The listing builds one solid part. Answer for the finished solid, in the listing's coordinates (mm). Face numbers are marked on the shaded views. Round coordinates to 2 decimals unless told otherwise and drop trailing zeros. Write each loop counter-clockwise with the first axis right and the second up, starting at its lowest first coordinate (ties: lowest second). Pieces come first, ordered by that corner, then holes. Notation, with made-up numbers: (30.25, 19) - (70.25, 19) arc R10 ccw to (70.25, 24) - close; hole circle Ø7 at (23.25, 71.5). An arc over 180 degrees is marked (long way). Answer as CSV lines item,"result". Start each with the question number.
Item 1: A cutting plane is placed at C-C on z = 65. Determine the outline of the cut face in (x, y), and give its area (3 significant figures).
Item 2: A cutting plane is placed at A-A on x = 0. Determine the outline of the cut face in (y, z), and give its area (3 significant figures).
Item 3: Straight lines are drawn through the part: line 1 along Y through (x, z) = (0, 61); line 2 along Y through (x, z) = (-1.5, 22). For each, find the intervals that lie inside material, in ascending order. Write a range as [from, to].
Item 4: Flat-ended cylindrical pins translate along their axes: pin 1 (3 mm diameter, centred on x = 8, y = 0.5, fed in from +Z); pin 2 (6 mm diameter, centred on y = 7, z = 55, fed in from -X); pin 3 (12 mm diameter, centred on x = 0.5, z = -16.5, fed in from +Y). Find the tip coordinate at first contact, or state that the pin passes through.
Item 5: For a pull along Y with two mould halves and no side action, classify the marked faces 1 and 2 as pulls with the +Y half, pulls with the -Y half, needs draft (parallel to the pull), parting line crosses it, or undercut.
Item 6: A cutting plane is placed at D-D on z = -5.5. Determine the outline of the cut face in (x, y), and give its area (3 significant figures).
Autodesk Inventor part; units mm, degrees
ref_plane "YZ Plane" through (0, 0, 0) normal (1, 0, 0) x (0, 1, 0)
ref_plane "XZ Plane" through (0, 0, 0) normal (0, 1, 0) x (-1, 0, 0)
ref_plane "XY Plane" through (0, 0, 0) normal (0, 0, 1) x (1, 0, 0)
sketch "Sketch1" plane through (0, 0, 0) normal (0, 0, 1) x (1, 0, 0)
  circle A0 centre (0, 0) radius 10
  circle A1 centre (0, 0) radius 11.2
  circle A2 centre (0, 0) radius 15.75
  dimension "d0" = 20
  dimension "d1" = 1.2
  dimension "d12" = 31.5
  dimension "d16" = 22.4
extrude "Extrusion1" add sketch "Sketch1" against normal blind 31.2 contours A0 | A1 | A2
extrude "Extrusion2" add sketch "Sketch1" along normal blind 80 contours A1
sketch "Sketch2" plane through (0, 0, 0) normal (0, 1, 0) x (-1, 0, 0)
  line L0 (-15.75, -31.2) -> (15.75, -31.2)
  line L1 (15.75, 0) -> (-15.75, 0) construction
  line L2 (-15.75, -31.2) -> (15.75, -31.2)
  line L3 (15.75, 0) -> (-15.75, 0)
  line L4 (15.75, -31.2) -> (15.75, 0) construction
  line L5 (-15.75, -31.2) -> (-15.75, 0) construction
  line L6 (-15.75, 0) -> (-15.75, -31.2) construction
  line L7 (15.75, -1.2) -> (-15.75, -1.2)
  line L8 (15.75, -1.2) -> (15.75, -31.2)
  line L9 (-15.75, -1.2) -> (-15.75, -31.2)
  line L10 (15.75, 0) -> (15.75, -31.2)
  arc A0 (15.75, -1.2) -> (12.9532, -3.1146) centre (15.75, -4.2) ccw
  arc A1 (-12.9532, -3.1146) -> (-15.75, -1.2) centre (-15.75, -4.2) ccw
  arc A2 (-2.7968, -29.2854) -> (2.7968, -29.2854) centre (0, -28.2) ccw
  line L11 (2.7968, -29.2854) -> (12.9532, -3.1146)
  line L12 (-12.9532, -3.1146) -> (-2.7968, -29.2854)
  line L13 (0, -31.2) -> (0, -1.2)
  line L14 (-11.2, 0) -> (-11.2, 80) construction
  line L15 (-15.75, 0) -> (-11.2, 4.55)
  line L16 (-11.2, 0) -> (-11.2, 80)
  line L17 (-11.2, 4.55) -> (-11.2, 0)
  line L18 (-11.2, 0) -> (-15.75, 0)
  point P0 (0, 0)
  dimension "d7" = 1.2
  dimension "d10" = 3
  dimension "d14" = 45
revolve "Revolution1" cut sketch "Sketch2" angle 360 about axis through (0, 0, -31.2) along (0, 0, 1) contours L9 A1 L12 A2 L0
revolve "Revolution2" add sketch "Sketch2" angle 360 about axis through (0, 0, -31.2) along (0, 0, 1) contours L3 L15 L16 | A2 L12 A1 L7 L13
sketch "Sketch3" plane through (0, 0, 0) normal (0, 0, 1) x (1, 0, 0)
  circle A0 centre (0, 0) radius 4.5
  dimension "d17" = 9
extrude "Extrusion4" add sketch "Sketch3" along normal blind 10
properties part number "Static Marker Barrel" material "ABS Plastic"
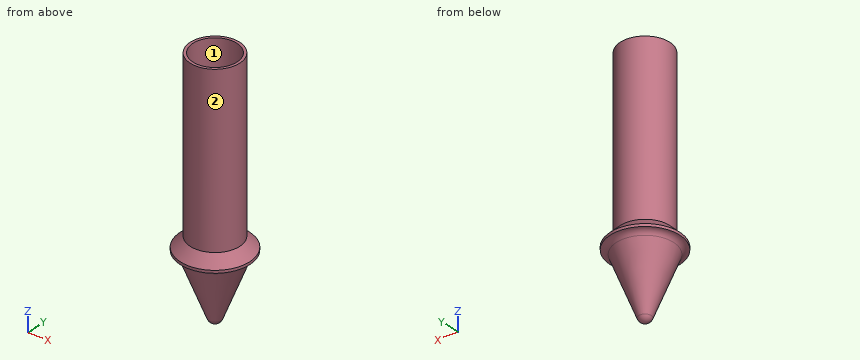
Geometry says:
1,outline,"circle Ø22.4 at (0, 0); hole circle Ø20 at (0, 0)"
1,area,"79.9 mm^2"
2,outline,"(-15.75, -1.2) arc R3 cw to (-12.95, -3.11) - (-2.8, -29.29) arc R3 ccw to (2.8, -29.29) - (12.95, -3.11) arc R3 cw to (15.75, -1.2) - (15.75, 0) - (11.2, 4.55) - (11.2, 80) - (10, 80) - (10, 0) - (4.5, 0) - (4.5, 10) - (-4.5, 10) - (-4.5, 0) - (-10, 0) - (-10, 80) - (-11.2, 80) - (-11.2, 4.55) - (-15.75, 0) - close"
2,area,"813 mm^2"
3,line 1,"y = [-11.2, -10], [10, 11.2]"
3,line 2,"y = [-11.1, -9.89], [9.89, 11.1]"
4,pin 1,"stops at z = 0"
4,pin 2,"stops at x = -10.46"
4,pin 3,"stops at y = 10.08"
5,face 1,"undercut"
5,face 2,"parting line crosses it"
6,outline,"circle Ø24.05 at (0, 0)"
6,area,"454 mm^2"
